Can you work these out from the model? Positions are in its coordinate system, mm. A direction names the side the tool comes from. Give positions to 0.01 mm unless a question says otherwise; leave off trailing zeros. Order: outer loops, then holes, each group sorted by start corner. A loop starts at its lowest first (then second) coordinate and runs counter-clockwise, first axis right, second up. Notation, with made-up numbers: (5.25, 6) - (46.25, 6) arc R16 cw to (46.25, 22) - close; hole circle Ø11 at (9.25, 79). An arc over 180 degrees is marked (long way). Answer as a JSON object with one key per item and string values.
```python
from build123d import *

# Parameters (mm, degrees)
CROQUIS1_W              = 45
CROQUIS1_H              = 115
SALIENTE_EXTRUIR1_DEPTH = 5
CROQUIS3_W              = 22.5
CROQUIS3_H              = 2
CORTAR_EXTRUIR2_DEPTH   = 5
REDONDEO1_R             = 3
CROQUIS4_W              = 2
CROQUIS4_H              = 8
CORTAR_EXTRUIR3_DEPTH   = 5
REDONDEO2_R             = 0.5


with BuildPart() as part:
    # Croquis1 → Saliente-Extruir1 (new body)
    with BuildSketch(Plane.XY):
        with Locations((0, -12.5)):
            Rectangle(CROQUIS1_W, CROQUIS1_H)
    extrude(amount=SALIENTE_EXTRUIR1_DEPTH)

    # Croquis3 → Cortar-Extruir2 (cut)
    with BuildSketch(Plane.XY.offset(5)):
        with Locations((11.25, -64)):
            Rectangle(CROQUIS3_W, CROQUIS3_H)
    extrude(amount=-CORTAR_EXTRUIR2_DEPTH, mode=Mode.SUBTRACT)

    # Redondeo1
    redondeo1_edges = [part.edges().sort_by_distance(p)[0] for p in [
        (-22.5, 45, 2.5),
        (-22.5, -70, 2.5),
        (22.5, 45, 2.5),
    ]]
    fillet(redondeo1_edges, radius=REDONDEO1_R)

    # Croquis4 → Cortar-Extruir3 (cut)
    with BuildSketch(Plane.XY.offset(5)):
        with Locations((0, 41)):
            Rectangle(CROQUIS4_W, CROQUIS4_H)
    extrude(amount=-CORTAR_EXTRUIR3_DEPTH, mode=Mode.SUBTRACT)

    # Redondeo2
    redondeo2_edges = [part.edges().sort_by_distance(p)[0] for p in [
        (0, -63, 2.5),
        (0, -65, 2.5),
        (22.5, -65, 2.5),
        (22.5, -63, 2.5),
        (22.5, -70, 2.5),
    ]]
    fillet(redondeo2_edges, radius=REDONDEO2_R)


solid = part.part
```
Q1. I'm going to push flat-ended pins straight in: pin 1 Ø0.8 at (y, z) = (-64, 3.5) entering from +X; pin 2 Ø1 at (x, z) = (0, 3.5) entering from +Y. Where does each tip first touch, or does it pass through?
Recorded:
{"pin 1": "stops at x = 0", "pin 2": "stops at y = 37"}
Q2. We'd pull the mould along X, two halves only. Please class faces 1 (the face through (-1, 41, 3)), 2 (the face through (21.6, 44.14, 2.54)), 3 (the face through (0, -12, 5)): released by +X, released by -X, zero draft, split by the parting line, or undercut.
Recorded:
{"face 1": "undercut", "face 2": "released by +X", "face 3": "zero draft"}
Q3. If we section it at A-A, the plane x = 3.5: Please give me the cut outline in (y, z).
Recorded:
{"outline": "(-70, 0) - (-65, 0) - (-65, 5) - (-70, 5) - close; (-63, 0) - (45, 0) - (45, 5) - (-63, 5) - close"}
Q4. I need wall thicknesses on L1, parallel to Y at x = 11.5, z = 2.7; L2, parallel to Y at x = 0.5, z = 3.65; L3, parallel to Y at x = -20.5, z = 2.1. Which ranges of each line are inside material? Lowest first, please.
Recorded:
{"L1": "y = -70 to -65, -63 to 45", "L2": "y = -70 to -65, -63 to 37", "L3": "y = -69.83 to 44.83"}
Q5. Which directions (+Z, -Z, +X, -X, +Y, -Y) give clear straight access to the entire face, cutting with the end or side of a thin tool? Please do faces 4 (the face through (11, -65, 3)), 5 (the face through (0, 37, 3)), 6 (the face through (22.5, -11, 2)).
Recorded:
{"face 4": "+Z, -Z, +X", "face 5": "+Z, -Z, +Y", "face 6": "+Z, -Z, +X, +Y, -Y"}
